```python
from build123d import *

# Parameters (mm, degrees)
F0_W     = 50.8
F0_H     = 31.75
F1_DEPTH = 25.4
F3_DEPTH = 12.7
F4_W     = 50.8
F4_H     = 21.5396340117
F5_DEPTH = 12.7
F6_W     = 10.3306490928
F6_H     = 21.5396340117
F7_DEPTH = 25.4
F9_DEPTH = 25.4


with BuildPart() as f1:
    # F0 (on Front) → F1 (new body)
    with BuildSketch(Plane.XZ):
        with Locations((25.4, 15.875)):
            Rectangle(F0_W, F0_H)
    extrude(amount=F1_DEPTH)

    # F2 (on face) → F3 (cut)
    with BuildSketch(Plane(origin=(0, 0, 0), x_dir=(-1, 0, 0), z_dir=(0, 1, 0))):
        Polygon((-50.8, 31.75), (-50.8, 15.875), (-38.1, 31.75), align=None)
    extrude(amount=-F3_DEPTH, mode=Mode.SUBTRACT)

    # F4 (on face) → F5 (cut)
    with BuildSketch(Plane.XZ.offset(25.4)):
        with Locations((25.4, 20.9801829942)):
            Rectangle(F4_W, F4_H)
    extrude(amount=-F5_DEPTH, mode=Mode.SUBTRACT)

    # F6 (on face) → F7 (join)
    with BuildSketch(Plane.XZ.offset(12.7)):
        with Locations((21.4760145172, 20.9801829942)):
            Rectangle(F6_W, F6_H)
    extrude(amount=F7_DEPTH)

    # F8 (on face) → F9 (cut)
    with BuildSketch(Plane(origin=(16.3106899709, 0, 0), x_dir=(0, -1, 0), z_dir=(-1, 0, 0))):
        Polygon((38.1, 31.75), (12.7, 31.75), (25.4, 10.2103659883), (38.1, 10.2103659883), align=None)
    extrude(amount=-F9_DEPTH, mode=Mode.SUBTRACT)


solid = f1.part
```
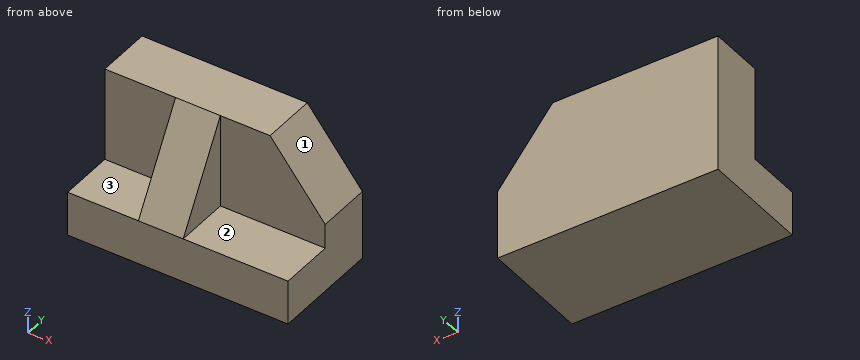
Model file for the job. Use its own axes, mm. Face numbers are marked on the shaded views. A direction names the side the tool comes from. Coordinates: 2 decimals unless noted, no trailing zeros. Write each loop counter-clockwise with the first axis right and the second up, starting at its lowest first coordinate (ties: lowest second). Pieces come first, ordered by that corner, then holes. Notation, with made-up numbers: (35, 48) - (44, 48) arc R26 cw to (44, 76) - close; hole circle Ø6 at (66, 39). An arc over 180 degrees is marked (long way). Use a Markdown table: item, result. Add a question column.
Item 1: 3-axis set-ups, long thin cutter, end or side, ignore diameter. For the marked faces 1, 2 and 3: which of +Z, -Z, +X, -X, +Y, -Y reach the whole face in a straight line?
Item 2: Drop flat-ended pins along their axis: pin 1 (1 mm diameter, centred on x = 31.5, z = 10.5, fed in from +Y); pin 2 (5 mm diameter, centred on x = 22, z = 24.5, fed in from -Y); pin 3 (2 mm diameter, centred on x = 33.5, z = 26, fed in from -Y); pin 4 (4 mm diameter, centred on x = 43.5, y = -20.5, fed in from +Z). Give the stop position or say it passes through.
Item 3: Band-saw the part on B-B, the plane z = 24. Write the cut outline in (x, y), and give its area (3 significant figures).
Item 4: Band-saw the part on C-C, the plane x = 21. Write the cut outline in (y, z), and give its area (3 significant figures).
Item 5: Drill centre lines: line 1 along Y through (x, z) = (47.5, 15.5); line 2 along Z through (x, y) = (33.5, -20); line 3 along X through (y, z) = (-18.5, 19). Where is each one in solid material? Low to high.
Item 6: Band-saw the part on A-A, the plane y = -1.5. Write the cut outline in (x, z) (3 decimals).
Item 7: Band-saw the part on D-D, the plane y = -20. Write the cut outline in (x, z), and give its area (3 significant figures).
A:
| question | item | result |
|---|---|---|
| 1 | face 1 | +Z, +X, +Y, -Y |
| 1 | face 2 | +Z, +X, -Y |
| 1 | face 3 | +Z, -X, -Y |
| 2 | pin 1 | stops at y = 0 |
| 2 | pin 2 | stops at y = -18.45 |
| 2 | pin 3 | stops at y = -12.7 |
| 2 | pin 4 | stops at z = 10.21 |
| 3 | outline | (0, -12.7) - (16.31, -12.7) - (16.31, -17.27) - (26.64, -17.27) - (26.64, -12.7) - (44.3, -12.7) - (44.3, 0) - (0, 0) - close |
| 3 | area | 610 mm² |
| 4 | outline | (-25.4, 0) - (0, 0) - (0, 31.75) - (-12.7, 31.75) - (-25.4, 10.21) - close |
| 4 | area | 670 mm² |
| 5 | line 1 | y = -12.7 to 0 |
| 5 | line 2 | z = 0 to 10.21 |
| 5 | line 3 | x = 16.31 to 26.64 |
| 6 | outline | (0, 0) - (50.8, 0) - (50.8, 15.875) - (38.1, 31.75) - (0, 31.75) - close |
| 7 | outline | (0, 0) - (50.8, 0) - (50.8, 10.21) - (26.64, 10.21) - (26.64, 19.37) - (16.31, 19.37) - (16.31, 10.21) - (0, 10.21) - close |
| 7 | area | 613 mm² |
